Source: CAD feature listing. Evaluate the final solid. Frame: model axes, mm. A direction names the side the tool comes from. Give positions to 0.01 mm unless a question says otherwise; leave off trailing zeros. Write each loop counter-clockwise with the first axis right and the second up, starting at its lowest first coordinate (ties: lowest second). Pieces come first, ordered by that corner, then holes. Notation, with made-up numbers: M 88.5,-26 L 141.5,-26 A11 cw 141.5,-10 Z; hole C 61,84.5 d7. An arc over 180 degrees is marked long. Use CSV: the item, a comma, the result in double quotes. Start each with the question number.
Autodesk Inventor part; units mm, degrees
ref_plane "YZ Plane" through (0, 0, 0) normal (1, 0, 0) x (0, 1, 0)
ref_plane "XZ Plane" through (0, 0, 0) normal (0, 1, 0) x (-1, 0, 0)
ref_plane "XY Plane" through (0, 0, 0) normal (0, 0, 1) x (1, 0, 0)
sketch "Sketch1" plane through (0, 0, 0) normal (0, 1, 0) x (-1, 0, 0)
  line L0 (-21, 22) -> (21, 22)
  line L1 (21, 22) -> (21, -22)
  line L2 (21, -22) -> (-21, -22)
  line L3 (-21, -22) -> (-21, 22)
  line L4 (-21, 22) -> (21, -22) construction
  line L5 (21, 22) -> (-21, -22) construction
  point P0 (0, 0)
  dimension "d0" = 42
  dimension "d1" = 44
extrude "wall2" add sketch "Sketch1" along normal blind 6.4
sketch "Sketch7" plane through (0, 6.4, 0) normal (0, 1, 0) x (1, 0, 0)
  line L0 (5, -22) -> (5, 22) construction
  line L1 (21, 22) -> (-21, 22)
  line L2 (-21, -22) -> (21, -22)
  line L3 (-21, 12) -> (21, 12) construction
  line L4 (21, -22) -> (21, 22)
  line L5 (-21, 22) -> (-21, -22)
  circle A0 centre (5, 12) radius 5.81
  point P0 (0, 0)
  dimension "d74" = 34
  dimension "d75" = 26
  dimension "d76" = 11.62
extrude "bigcircle" cut sketch "Sketch7" against normal blind 6.4 contours A0
sketch "Sketch8" plane through (0, 6.4, 0) normal (0, 1, 0) x (1, 0, 0)
  line L0 (-21, -22) -> (-21, 22)
  line L1 (-21, 12) -> (21, 12) construction
  line L2 (21, 22) -> (21, -22)
  line L3 (5, 22) -> (5, -22) construction
  line L4 (21, -22) -> (21, 22)
  line L5 (21, 22) -> (-21, 22)
  line L6 (-21, -22) -> (21, -22)
  circle A0 centre (-1, 12) radius 2.96
  point P0 (0, 0)
  dimension "d81" = 26
  dimension "d82" = 34
  dimension "d83" = 5.92
  dimension "d84" = 6
extrude "smallcircle" cut sketch "Sketch8" against normal blind 6.4 contours A0
fillet "Fillet4" radius 2 2 edges at (-0.0829, 3.2, -9.1857) (-0.0829, 3.2, -14.8143)
fillet_without_effect "Fillet5"
fillet "Fillet6" radius 2 1 edges at (-21, 3.2, -22)
fillet "Fillet7" radius 2 1 edges at (21, 3.2, -22)
fillet "Fillet8" radius 2 1 edges at (-21, 3.2, 22)
fillet "Fillet9" radius 2 1 edges at (21, 3.2, 22)
sketch "Sketch9" plane through (0, 6.4, 0) normal (0, 1, 0) x (1, 0, 0)
  line L0 (11.31, 17.1525) -> (11.31, -6.1616) construction
  line L1 (10.81, 14.2171) -> (10.81, 9.0836) construction
  arc A0 (0.512, 8.3102) -> (0.512, 15.6898) centre (5, 12) ccw
  line L2 (-21, 12) -> (18.6779, 12) construction
  line L3 (11.31, 9) -> (17.31, 9)
  line L4 (17.31, 9) -> (17.31, 15)
  line L5 (17.31, 15) -> (11.31, 15)
  line L6 (11.31, 15) -> (11.31, 9)
  line L7 (11.31, 9) -> (17.31, 15) construction
  line L8 (17.31, 9) -> (11.31, 15) construction
  line L9 (-21, 20) -> (-21, -20)
  line L10 (-18.49, 15) -> (-12.49, 15)
  line L11 (-12.49, 15) -> (-12.49, 9)
  line L12 (-12.49, 9) -> (-18.49, 9)
  line L13 (-18.49, 9) -> (-18.49, 15)
  line L14 (-18.49, 15) -> (-12.49, 9) construction
  line L15 (-12.49, 15) -> (-18.49, 9) construction
  point P0 (0, 0)
  point P1 (14.31, 12)
  point P2 (-15.49, 12)
  dimension "d93" = 0.5
  dimension "d94" = 6
  dimension "d95" = 23.3
extrude "Extrusion7" add sketch "Sketch9" along normal blind 4
equation "\"d0\" = wallw"
equation "\"d1\" = wallh"
equation "\"d72\" = wall2_thick"
equation "\"d74\" = distancefrombottom"
equation "\"d75\" = distancefromleft"
equation "\"d76\" = servobigcircledia"
equation "\"d79\" = wall2_thick"
equation "\"d81\" = distancefromleft"
equation "\"d82\" = distancefrombottom"
equation "\"d83\" = servosmallcircledia"
equation "\"d85\" = wall2_thick"
equation "\"d89\" = cornerrad"
equation "\"d90\" = cornerrad"
equation "\"d91\" = cornerrad"
equation "\"d92\" = cornerrad"
equation "\"d94\" = servomountsquare"
equation "\"d96\" = servomounth"
equation "\"printer3dtolerance\" = 0.12"
equation "\"wallw\" = 42"
equation "\"wallh\" = 44"
equation "\"cornerrad\" = 2"
equation "\"baseextra\" = 2"
equation "\"wall1_thick\" = 8"
equation "\"wall2_thick\" = 6.4"
equation "\"wall3_thick\" = 4"
equation "\"wall1slot\" = 8.12"
equation "\"wall2slot\" = 6.52"
equation "\"wall3slot\" = 4.12"
equation "\"gap2\" = 28"
equation "\"baseh\" = 79.12"
equation "\"basew\" = 44"
equation "\"base_thick\" = 6"
equation "\"base_slots_depth\" = 4"
equation "\"servomounth\" = 4"
equation "\"servosmallcircledia\" = 5.92"
equation "\"servomountsquare\" = 6"
equation "\"servobigcircledia\" = 11.62"
equation "\"servo9gw\" = 22.8"
equation "\"distancefromleft\" = 26"
equation "\"servopolygonl\" = 5.92"
equation "\"servopolygonr\" = 6.12"
equation "\"distancefrombottom\" = 34"
equation "\"d49\" = distancefrombottom"
equation "\"adapterh\" = 16"
equation "\"wall3slotd\" = 2"
equation "\"adapterw\" = 32"
equation "\"wall3slotd_1\" = 2"
equation "\"wall3slotw\" = 36"
properties part number "wall-middle" material "Wood (Oak)"
1. Access query for faces 1 (the flat face through (-18.49, 8, -12)), 2 (the flat face through (-16, 8, -15)), 3 (the flat face through (14, 8, -9)). Directions: +Z, -Z, +X, -X, +Y, -Y. A direction counts if a zero-diameter tool reaches every point of the face in a straight line with its end or side. Return the directions, or none.
2. First-contact query: pin 1 (1.2 mm diameter, centred on y = 9, z = -11.5, fed in from -X); pin 2 (3 mm diameter, centred on x = 13, y = 8.5, fed in from +Z); pin 3 (1.2 mm diameter, centred on x = 14.5, y = 8, fed in from -Z). Flat tips, straight axial feed; report the tip coordinate or a pass-through.
3. Section D-D on x = 12. Return loops of the section in (y, z).
4. Section A-A on z = -12. Return loops of the section in (x, y).
5. Section C-C on x = 5. Return loops of the section in (y, z).
6. Line query: probe 1 along Z at (x, y) = (5, 3.75); probe 2 along X at (y, z) = (8.25, -14); probe 3 along Y at (x, z) = (3.5, -3). Output: solid intervals per line, ascending.
7. Section B-B on y = 8.5. Return loops of the section in (x, z), then the cut area to 3 significant figures.
Resolved:
1,face 1,"+Z, -Z, -X, +Y"
1,face 2,"-Z, +X, -X, +Y"
1,face 3,"+Z, +X, -X, +Y"
2,pin 1,"stops at x = -18.49"
2,pin 2,"stops at z = -9"
2,pin 3,"stops at z = -15"
3,outline,"M 0,-22 L 6.4,-22 L 6.4,-15 L 10.4,-15 L 10.4,-9 L 6.4,-9 L 6.4,22 L 0,22 Z"
4,outline,"M -21,0 L -3.96,0 L -3.96,6.4 L -12.49,6.4 L -12.49,10.4 L -18.49,10.4 L -18.49,6.4 L -21,6.4 Z; M 10.81,0 L 21,0 L 21,6.4 L 17.31,6.4 L 17.31,10.4 L 11.31,10.4 L 11.31,6.4 L 10.81,6.4 Z"
5,outline,"M 0,-22 L 6.4,-22 L 6.4,-17.81 L 0,-17.81 Z; M 0,-6.19 L 6.4,-6.19 L 6.4,22 L 0,22 Z"
6,probe 1,"z = -22 to -17.81, -6.19 to 22"
6,probe 2,"x = -18.49 to -12.49, 11.31 to 17.31"
6,probe 3,"y = 0 to 6.4"
7,outline,"M -18.49,-15 L -12.49,-15 L -12.49,-9 L -18.49,-9 Z; M 11.31,-15 L 17.31,-15 L 17.31,-9 L 11.31,-9 Z"
7,area,"72.0 mm2"
